Input: part model. Units: mm. Frame: model coordinates. A direction names the side the tool comes from. Round coordinates to 2 decimals unless told otherwise and drop trailing zeros. Write each loop counter-clockwise with the first axis right and the second up, starting at its lowest first coordinate (ties: lowest second). Pieces come first, ordered by that corner, then holes. Notation, with made-up numbers: M 61,-28.5 L 93,-28.5 A32 cw 93,3.5 Z; hole C 69.5,-36 d11. An arc over 180 degrees is marked long. Write each question's results on one line, items separated by ' | '. Start each with the question number.
```python
from build123d import *
from OCP.BRepFilletAPI import BRepFilletAPI_MakeChamfer

# Parameters (mm, degrees)
SKETCH_1_R                         = 13
EXTRUDE_1_DEPTH                    = 10
SKETCH_2_R                         = 2.7
CUT_EXTRUDE_1_DEPTH                = 5
PATTERN_CIRCULAR_1_COUNT           = 3
PATTERN_CIRCULAR_1_COPY_1_SKETCH_R = 2.7
PATTERN_CIRCULAR_1_COPY_1_DEPTH    = 5
PATTERN_CIRCULAR_1_COPY_2_SKETCH_R = 2.7
PATTERN_CIRCULAR_1_COPY_2_DEPTH    = 5
SKETCH_3_R                         = 2.7
SKETCH_3_R_2                       = 2.699999999999997
SKETCH_3_R_3                       = 2.700000000000001
CUT_EXTRUDE_2_DEPTH                = 5
SKETCH_4_R                         = 1.5000000000000009
SKETCH_4_R_2                       = 1.5000000000000042
CUT_EXTRUDE_3_DEPTH                = 61.95246780158357
CUT_EXTRUDE_5_DEPTH                = 61.95246780158357
SKETCH_7_R                         = 3.2
SKETCH_7_R_2                       = 3.1999999999999984
CUT_EXTRUDE_6_DEPTH                = 8
CHAMFER_2_SIZE                     = 1.4
FILLET_2_R                         = 2
CHAMFER_3_SIZE                     = 1.4
SKETCH_9_R                         = 1.8000000000000005
SKETCH_9_R_2                       = 1.7999999999999987
SKETCH_9_R_3                       = 1.8
CUT_EXTRUDE_8_DEPTH                = 60.81513460321006
SKETCH_10_R                        = 1.8000000000000014
CUT_EXTRUDE_9_DEPTH                = 10
PATTERN_CIRCULAR_2_COUNT           = 3
PATTERN_CIRCULAR_2_COPY_1_SKETCH_R = 1.8000000000000014
PATTERN_CIRCULAR_2_COPY_1_DEPTH    = 10
PATTERN_CIRCULAR_2_COPY_2_SKETCH_R = 1.8000000000000014
PATTERN_CIRCULAR_2_COPY_2_DEPTH    = 10
SKETCH_11_R                        = 1.5000000000000009
CUT_EXTRUDE_10_DEPTH               = 61.43881474350847
SKETCH_12_R                        = 2.6999999999999993
CUT_EXTRUDE_11_DEPTH               = 61.140255466701646
CUT_EXTRUDE_12_DEPTH               = 61.43881474350847
CHAMFER_4_SIZE                     = 3
CHAMFER_4_SIZE2                    = 2.6704845794861627
CHAMFER_4_SIZE2_2                  = 2.670484579486165


with BuildPart() as part:
    # 草圖1 → 填料-伸長1 (new body)
    with BuildSketch(Plane.XY):
        Polygon((-20.49999999999998, 39.999999999999986), (20.49999999999997, 39.99999999999999), (20.499999999999982, 29.999999999999993), (36.23076211353136, 2.753520777584056), (44.891016151375794, -2.2464792224159686), (24.39101615137583, -37.753520777577926), (15.730762113531437, -32.75352077757793), (-15.730762113531332, -32.753520777577926), (-24.391016151375762, -37.75352077757796), (-44.891016151375766, -2.2464792224160335), (-36.23076211353138, 2.7535207775839847), (-20.49999999999998, 29.999999999999936), align=None)
        Circle(SKETCH_1_R, mode=Mode.SUBTRACT)
    extrude(amount=EXTRUDE_1_DEPTH)

    # 草圖2 → 除料-伸長1 (cut)
    with BuildSketch(Plane.ZY.offset(20.49999999999998)):
        with Locations((5, 34.999999999999964)):
            Circle(SKETCH_2_R)
    cut_extrude_1 = extrude(amount=-CUT_EXTRUDE_1_DEPTH, mode=Mode.SUBTRACT)

    # 鏡射1: 除料-伸長1 across plane
    add(cut_extrude_1.mirror(Plane(origin=(0, 0, 0), x_dir=(0, 0, 1), z_dir=(1, 0, 0))), mode=Mode.SUBTRACT)

    # 環狀複製排列1: 除料-伸長1 ×3 about axis
    pattern_circular_1_axis = Axis((1.45e-15, -5e-16, 0), (0, 0, 1))
    for i in range(1, PATTERN_CIRCULAR_1_COUNT):
        add(cut_extrude_1.rotate(pattern_circular_1_axis, i * 360 / PATTERN_CIRCULAR_1_COUNT), mode=Mode.SUBTRACT)

    # 環狀複製排列1 copy 1 sketch → 環狀複製排列1 copy 1 (cut)
    with BuildSketch(Plane(origin=(-10.249999999999982, 17.75352077758097, 0), x_dir=(0, 0, 1), z_dir=(-0.4999999999999998, 0.8660254037844387, 0))):
        with Locations((5, -34.999999999999964)):
            Circle(PATTERN_CIRCULAR_1_COPY_1_SKETCH_R)
    extrude(amount=-PATTERN_CIRCULAR_1_COPY_1_DEPTH, mode=Mode.SUBTRACT)

    # 環狀複製排列1 copy 2 sketch → 環狀複製排列1 copy 2 (cut)
    with BuildSketch(Plane(origin=(-10.249999999999996, -17.753520777580967, 0), x_dir=(0, 0, 1), z_dir=(-0.5000000000000004, -0.8660254037844384, 0))):
        with Locations((5, -34.999999999999964)):
            Circle(PATTERN_CIRCULAR_1_COPY_2_SKETCH_R)
    extrude(amount=-PATTERN_CIRCULAR_1_COPY_2_DEPTH, mode=Mode.SUBTRACT)

    # 草圖3 → 除料-伸長2 (cut)
    with BuildSketch(Plane(origin=(0, 0, 10), x_dir=(-1, 0, 0), z_dir=(0, 0, -1))):
        with Locations((2.04439e-12, 18)):
            Circle(SKETCH_3_R)
        with Locations((15.588457268121106, -9.000000000000483)):
            Circle(SKETCH_3_R_2)
        with Locations((-15.588457268118686, -8.999999999999522)):
            Circle(SKETCH_3_R_3)
    extrude(amount=CUT_EXTRUDE_2_DEPTH, mode=Mode.SUBTRACT)

    # 草圖4 → 除料-伸長3 (cut, through all)
    with BuildSketch(Plane(origin=(0, 0, 0), x_dir=(-1, 0, 0), z_dir=(0, 0, -1))):
        with Locations((22, -12)):
            Circle(SKETCH_4_R)
        with Locations((21.999999999999986, 12.000000000000002)):
            Circle(SKETCH_4_R)
        with Locations(Location((-21.999999999999986, 12.000000000000002, 0), (0, 0, 180))):
            Circle(SKETCH_4_R_2)
        with Locations(Location((-22, -12, 0), (0, 0, 180))):
            Circle(SKETCH_4_R)
    extrude(amount=-CUT_EXTRUDE_3_DEPTH, mode=Mode.SUBTRACT)

    # 草圖6 → 除料-伸長5 (cut, through all)
    with BuildSketch(Plane.XY.offset(10)):
        with BuildLine():
            Line((3, 34), (3.0000000000000013, 26))
            ThreePointArc((3.0000000000000013, 26), (1.8e-16, 23), (-2.9999999999999996, 26))
            Line((-2.9999999999999996, 26), (-3.000000000000001, 34))
            ThreePointArc((-3.000000000000001, 34), (-6e-17, 37), (3, 34))
        make_face()
    extrude(amount=-CUT_EXTRUDE_5_DEPTH, mode=Mode.SUBTRACT)

    # 草圖7 → 除料-伸長6 (cut)
    with BuildSketch(Plane.XY.offset(10)):
        with Locations((-13.000000000000004, 24)):
            Circle(SKETCH_7_R)
        with Locations(Location((12.999999999999996, 24.000000000000004, 0), (0, 0, 180))):
            Circle(SKETCH_7_R_2)
    extrude(amount=-CUT_EXTRUDE_6_DEPTH, mode=Mode.SUBTRACT)

    # 導角2
    chamfer_2_edges = [part.edges().sort_by_distance(p)[0] for p in [
        (-34.641016151375766, -19.999999999996998, 10),
        (-3.55e-15, 39.999999999999986, 0),
        (34.64101615137581, -19.999999999996945, 0),
        (-34.641016151375766, -19.999999999996998, 0),
        (34.64101615137581, -19.999999999996945, 10),
        (-3.55e-15, 39.999999999999986, 10),
    ]]
    chamfer(chamfer_2_edges, length=CHAMFER_2_SIZE)

    # 圓角2
    fillet_2_edges = [part.edges().sort_by_distance(p)[0] for p in [
        (39.95467134980447, 0.6035207775840439, 10),
        (39.95467134980447, 0.6035207775840439, 0),
        (20.49999999999998, 34.3, 10),
        (20.49999999999998, 34.29999999999999, 0),
        (-20.49999999999998, 34.29999999999996, 10),
        (-20.49999999999998, 34.29999999999996, 0),
        (-39.95467134980447, 0.6035207775839742, 10),
        (-39.95467134980447, 0.603520777583975, 0),
        (-19.454671349804443, -34.903520777577945, 10),
        (-19.454671349804443, -34.903520777577945, 0),
        (19.45467134980452, -34.903520777577924, 10),
        (19.45467134980452, -34.903520777577924, 0),
        (36.23076211353136, 2.753520777584056, 5),
        (28.36538105676567, 16.376760388792025, 10),
        (20.499999999999982, 29.999999999999993, 5),
        (28.36538105676567, 16.376760388792025, 0),
        (-20.49999999999998, 29.999999999999936, 5),
        (-28.365381056765678, 16.376760388791958, 10),
        (-36.23076211353138, 2.7535207775839847, 5),
        (-28.365381056765678, 16.376760388791958, 0),
        (-15.730762113531332, -32.753520777577926, 5),
        (5.329e-14, -32.75352077757793, 10),
        (15.730762113531437, -32.75352077757793, 5),
        (5.329e-14, -32.75352077757793, 0),
    ]]
    fillet(fillet_2_edges, radius=FILLET_2_R)

    # 導角3
    chamfer_3_edges = [part.edges().sort_by_distance(p)[0] for p in [
        (20.476835451633185, 39.99999999999999, 8.30351539856506),
        (20.476835451633185, 39.99999999999999, 1.6964846014349406),
        (20.49999999999997, 39.99999999999999, 5),
        (44.8794338771924, -2.266540309768801, 8.303515398565063),
        (44.8794338771924, -2.266540309768801, 1.6964846014349366),
        (44.891016151375794, -2.2464792224159686, 5),
        (24.402598425559223, -37.73345969022509, 8.303515398565105),
        (24.402598425559223, -37.73345969022509, 1.6964846014348944),
        (24.39101615137583, -37.753520777577926, 5),
        (-24.402598425559155, -37.73345969022514, 8.30351539856507),
        (-24.402598425559155, -37.73345969022514, 1.6964846014349295),
        (-24.391016151375762, -37.75352077757796, 5),
        (-44.879433877192376, -2.2665403097688666, 8.303515398565079),
        (-44.879433877192376, -2.2665403097688643, 1.6964846014349226),
        (-44.891016151375766, -2.2464792224160335, 5),
        (-20.476835451633193, 39.999999999999986, 8.303515398565068),
        (-20.476835451633193, 39.999999999999986, 1.696484601434932),
        (-20.49999999999998, 39.999999999999986, 5),
    ]]
    chamfer(chamfer_3_edges, length=CHAMFER_3_SIZE - 0.0001)  # a hair under: the kernel refuses the full size

    # 草圖9 → 除料-伸長8 (cut, through all)
    with BuildSketch(Plane.XY.offset(5)):
        with Locations((15.588457268118686, -8.999999999999522)):
            Circle(SKETCH_9_R)
        with Locations((-15.58845726811887, -8.999999999999208)):
            Circle(SKETCH_9_R_2)
        with Locations((1.8019e-13, 17.999999999998714)):
            Circle(SKETCH_9_R_3)
    extrude(amount=-CUT_EXTRUDE_8_DEPTH, mode=Mode.SUBTRACT)

    # 草圖10 → 除料-伸長9 (cut)
    with BuildSketch(Plane.ZY.offset(15.499999999999979)):
        with Locations((5, 34.999999999999964)):
            Circle(SKETCH_10_R)
    cut_extrude_9 = extrude(amount=-CUT_EXTRUDE_9_DEPTH, mode=Mode.SUBTRACT)

    # 鏡射2: 除料-伸長9 across plane
    add(cut_extrude_9.mirror(Plane(origin=(0, 0, 0), x_dir=(0, 0, 1), z_dir=(1, 0, 0))), mode=Mode.SUBTRACT)

    # 環狀複製排列2: 除料-伸長9 ×3 about axis
    pattern_circular_2_axis = Axis((5.8e-16, 1e-15, 0), (0, 0, 1))
    for i in range(1, PATTERN_CIRCULAR_2_COUNT):
        add(cut_extrude_9.rotate(pattern_circular_2_axis, i * 360 / PATTERN_CIRCULAR_2_COUNT), mode=Mode.SUBTRACT)

    # 環狀複製排列2 copy 1 sketch → 環狀複製排列2 copy 1 (cut)
    with BuildSketch(Plane(origin=(-7.749999999999984, 13.423393758658783, 0), x_dir=(0, 0, 1), z_dir=(-0.4999999999999998, 0.8660254037844387, 0))):
        with Locations((5, -34.999999999999964)):
            Circle(PATTERN_CIRCULAR_2_COPY_1_SKETCH_R)
    extrude(amount=-PATTERN_CIRCULAR_2_COPY_1_DEPTH, mode=Mode.SUBTRACT)

    # 環狀複製排列2 copy 2 sketch → 環狀複製排列2 copy 2 (cut)
    with BuildSketch(Plane(origin=(-7.7499999999999964, -13.423393758658774, 0), x_dir=(0, 0, 1), z_dir=(-0.5000000000000004, -0.8660254037844384, 0))):
        with Locations((5, -34.999999999999964)):
            Circle(PATTERN_CIRCULAR_2_COPY_2_SKETCH_R)
    extrude(amount=-PATTERN_CIRCULAR_2_COPY_2_DEPTH, mode=Mode.SUBTRACT)

    # 草圖11 → 除料-伸長10 (cut, through all)
    with BuildSketch(Plane(origin=(0, 0, 0), x_dir=(-1, 0, 0), z_dir=(0, 0, -1))):
        with Locations((24, -20.999999999999996)):
            Circle(SKETCH_11_R)
        with Locations((-24, -20.999999999999996)):
            Circle(SKETCH_11_R)
        Polygon((-21, -15), (21, -15), (20.999999999999996, -27), (-20.999999999999996, -27), align=None)
    extrude(amount=-CUT_EXTRUDE_10_DEPTH, mode=Mode.SUBTRACT)

    # 草圖12 → 除料-伸長11 (cut, through all)
    with BuildSketch(Plane.XY.offset(2)):
        with Locations((-13.000000000000004, 24)):
            Circle(SKETCH_12_R)
        with Locations((12.999999999999996, 24.000000000000004)):
            Circle(SKETCH_12_R)
    extrude(amount=-CUT_EXTRUDE_11_DEPTH, mode=Mode.SUBTRACT)

    # 草圖13 → 除料-伸長12 (cut, through all)
    with BuildSketch(Plane.XY.offset(10)):
        Polygon((-13.000000000000002, 0), (-11, -14.999999999999996), (10.999999999999986, -15.000000000000007), (13.000000000000002, -1.203e-14), align=None)
    extrude(amount=-CUT_EXTRUDE_12_DEPTH, mode=Mode.SUBTRACT)

    # 導角4: one chamfer whose edges measure the first distance from different faces: ONE call of the kernel's chamfer builder (chamfer() names one face for all edges)
    chamfer_4_edges_1 = [part.edges().sort_by_distance(p)[0] for p in [
        (10.999999999999986, -15.000000000000007, 5),
    ]]
    chamfer_4_side_1 = [part.faces().sort_by_distance(p)[0] for p in [
        (15.999999999999993, -15, 5),
    ]]
    chamfer_4_edges_2 = [part.edges().sort_by_distance(p)[0] for p in [
        (-11, -14.999999999999996, 5),
    ]]
    chamfer_4_side_2 = [part.faces().sort_by_distance(p)[0] for p in [
        (-11.772925764192141, -9.203056768558943, 5),
    ]]
    chamfer_4 = BRepFilletAPI_MakeChamfer(part.part.solid().wrapped)
    for e in chamfer_4_edges_1:
        chamfer_4.Add(CHAMFER_4_SIZE, CHAMFER_4_SIZE2, e.wrapped, chamfer_4_side_1[0].wrapped)  # the first distance lies on this face
    for e in chamfer_4_edges_2:
        chamfer_4.Add(CHAMFER_4_SIZE, CHAMFER_4_SIZE2_2, e.wrapped, chamfer_4_side_2[0].wrapped)  # the first distance lies on this face
    add(Compound.cast(chamfer_4.Shape()), mode=Mode.REPLACE)


solid = part.part
```
1. Line query: L1, parallel to Y at x = 24, z = 4.75; L2, parallel to X at y = -7, z = 4.5; L3, parallel to Y at x = 18.45, z = 5. Output: solid intervals per line, ascending. Write a range as from..to.
2. Cut plane A-A on x = 0. Output: boundary loops of the cut face in (y, z), and give its area (3 significant figures).
3. Cut plane B-B on y = -9. Give the number of separate pieces and of enclosed holes in the cut face, and give its area (3 significant figures).
4. Contact query for flat-ended pins moving along their axis: P1, Ø5, axis at x = -22, y = 12, coming from the +Z side; P2, Ø3, axis at y = 35, z = 5, coming from the +X side; P3, Ø3, axis at y = 34.5, z = 4.5, coming from the -X side; P4, Ø6, axis at y = 35, z = 5, coming from the -X side. Output: stop coordinate, or through.
5. Draft query along X for faces 1 (the face through (-10.57, 33.243, 4.61)), 2 (the face through (-27.765, 16.276, 9.399)), 3 (the face through (-13.598, -7.175, 7.535)), 4 (the face through (17.731, -10.643, 7.535)). Return one class per face: +X half, -X half, draft (parallel to the pull), parting line (faces both ways), or undercut.
6. Access query for faces 5 (the face through (19.9, -34.5, 9.4)), 6 (the face through (21, -21, 5)), 7 (the face through (-11.28, 26.7, 6.06)). Directions: +Z, -Z, +X, -X, +Y, -Y. A direction counts if a zero-diameter tool reaches every point of the face in a straight line with its end or side. Return the directions, or none.
Answers follow:
1) L1: y = -36.83..-33.81, -24.87..-22.5, -19.5..23.94 | L2: x = -42.15..-38.37, -34.38..-12.07, 12.07..34.38, 38.37..42.15 | L3: y = -32.64..-27, -15..32.3, 37.7..40
2) outline: M -32.75,2 A2 ccw -30.75,0 L -27,0 L -27,10 L -30.75,10 A2 ccw -32.75,8 Z; M 13,0 L 16.2,0 L 16.2,5 L 15.3,5 L 15.3,10 L 13,10 Z; M 19.8,0 L 23,0 L 23,10 L 20.7,10 L 20.7,5 L 19.8,5 Z; M 37,0 L 38.6,0 L 40,1.4 L 40,8.6 L 38.6,10 L 37,10 Z | area: 139 mm2
3) separate pieces: 4 | enclosed holes: 2 | area: 466 mm2
4) P1: stops at z = 10 | P2: stops at x = 5.5 | P3: stops at x = -15.5 | P4: stops at x = -20.5
5) face 1: draft | face 2: -X half | face 3: undercut | face 4: undercut
6) face 5: +Z, -Y | face 6: +Z, -Z | face 7: +Z
